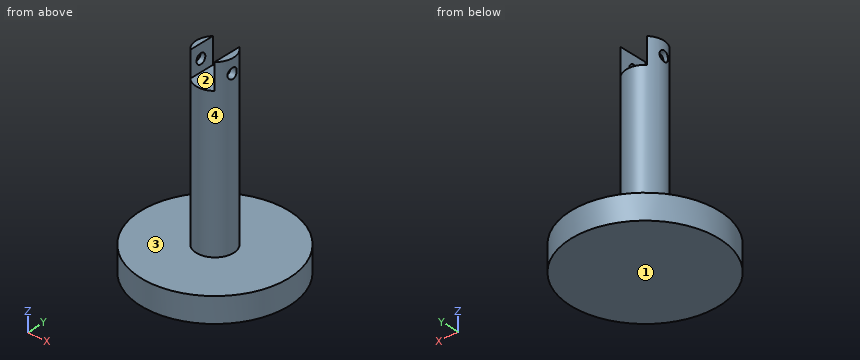
```python
from build123d import *

# Parameters (mm, degrees)
F0_R     = 75.4315959701
F1_DEPTH = 25.4
F10_R    = 19.05
F2_DEPTH = 203.2
F4_DEPTH = 26.25509
F5_R     = 5.3383463792
F6_DEPTH = 25.4
F7_R     = 5.1969918097
F8_DEPTH = 22.39609
F9_DEPTH = 72.38519


# Not quite as in the source:
# - a feature names something its author has since deleted; it is built from what else it names


with BuildPart() as f1:
    # F0 (on Top) → F1 (new body)
    with BuildSketch(Plane.XY):
        Circle(F0_R)
    extrude(amount=F1_DEPTH)

    # F10 (on Top) → F2 (join)
    with BuildSketch(Plane.XY):
        Circle(F10_R)
    extrude(amount=F2_DEPTH)

    # F3 (on face) → F4 (cut)
    with BuildSketch(Plane.XY.offset(203.2)):
        with BuildLine():
            ThreePointArc((12.2368524888, 14.6000664782), (-0.9386041951, 19.026863172), (-13.6144, 13.3248119176))
            Line((-13.6144, 13.3248119176), (-13.6144, -13.3248119176))
            ThreePointArc((-13.6144, -13.3248119176), (-0.9386041951, -19.026863172), (12.2368524888, -14.6000664782))
            Line((12.2368524888, -14.6000664782), (12.2368524888, 14.6000664782))
        make_face()
    extrude(amount=-F4_DEPTH, mode=Mode.SUBTRACT)

    # F5 (on face) → F6 (cut)
    with BuildSketch(Plane.YZ.offset(-13.6144)):
        with Locations((-189.9197250605, 0)):
            Circle(F5_R)
    extrude(amount=-F6_DEPTH, mode=Mode.SUBTRACT)

    # F7 (on face) → F8 (cut)
    with BuildSketch(Plane.YZ.offset(-13.6144)):
        with Locations((-0.8483366109, 189.2552375793)):
            Circle(F7_R)
    extrude(amount=-F8_DEPTH, mode=Mode.SUBTRACT)

    # F7 (on face) → F9 (cut)
    with BuildSketch(Plane.YZ.offset(-13.6144)):
        with Locations((-0.8483366109, 189.2552375793)):
            Circle(F7_R)
    extrude(amount=F9_DEPTH, mode=Mode.SUBTRACT)


solid = f1.part
```
Geometry: final body of the model. Coordinates: model frame, mm. Face numbers are marked on the shaded views. A direction names the side the tool comes from. Coordinates: 2 decimals unless noted, no trailing zeros. Order: outer loops, then holes, each group sorted by start corner. A loop starts at its lowest first (then second) coordinate and runs counter-clockwise, first axis right, second up. Notation, with made-up numbers: (68.25, -3) - (73.25, -3) arc R32 cw to (73.25, 29) - close; hole circle Ø1 at (-3.75, 10). An arc over 180 degrees is marked (long way). Write each question's results on one line, items separated by ' | '.
1) Section D-D, the plane y = 42. Return loops of the section in (x, z).
Results list:
outline: (-62.66, 0) - (62.66, 0) - (62.66, 25.4) - (-62.66, 25.4) - close
2) Pin query (flat end, axial travel): pin 1 (8 mm diameter, centred on y = 2, z = 195, fed in from +X); pin 2 (1 mm diameter, centred on x = -38, y = 8.5, fed in from -Z); pin 3 (12 mm diameter, centred on y = -0.85, z = 189.26, fed in from -X); pin 4 (6 mm diameter, centred on x = -55.5, y = 49.5, fed in from +Z). Return the tip coordinate at first contact, or that it passes through.
Results list:
pin 1: x = 19.05 | pin 2: z = 0 | pin 3: x = -19.05 | pin 4: z = 25.4
3) Set-up query: the marked faces 1 and 2. Return all of +Z, -Z, +X, -X, +Y, -Y with unobstructed straight access to the full face (end or side cutting, diameter ignored); none if empty.
Results list:
face 1: -Z, +X, -X, +Y, -Y | face 2: +Z, +Y, -Y
4) Section C-C, the plane z = 106. Return loops of the section in (x, y), plus the area to 3 significant figures.
Results list:
outline: circle Ø38.1 at (0, 0) | area: 1,140 mm^2
5) Line query: line 1 (Z direction, x = 44.5, y = 45); line 2 (Z direction, x = 7, y = -16.5); line 3 (X direction, y = 1, z = 102.5). Output: solid intervals per line, ascending. Write a range as from..to.
Results list:
line 1: 0..25.4 | line 2: 0..176.94 | line 3: -19.02..19.02
6) Pull-direction query (Y, two-part tool) for the marked faces 3 and 4; classes: pulls with the +Y half, pulls with the -Y half, needs draft (parallel to the pull), parting line crosses it, or undercut.
Results list:
face 3: needs draft | face 4: parting line crosses it
7) Section A-A, the plane y = 0. Return loops of the section in (x, z), plus the area to 3 significant figures.
Results list:
outline: (-75.43, 0) - (75.43, 0) - (75.43, 25.4) - (19.05, 25.4) - (19.05, 184.13) - (12.24, 184.13) - (12.24, 176.94) - (-13.61, 176.94) - (-13.61, 184.13) - (-19.05, 184.13) - (-19.05, 25.4) - (-75.43, 25.4) - close; (-19.05, 194.38) - (-13.61, 194.38) - (-13.61, 203.2) - (-19.05, 203.2) - close; (12.24, 194.38) - (19.05, 194.38) - (19.05, 203.2) - (12.24, 203.2) - close | area: 9,800 mm^2
8) Section B-B, the plane x = 0. Return loops of the section in (y, z), plus the area to 3 significant figures.
Results list:
outline: (-75.43, 0) - (75.43, 0) - (75.43, 25.4) - (19.05, 25.4) - (19.05, 176.94) - (-19.05, 176.94) - (-19.05, 25.4) - (-75.43, 25.4) - close | area: 9,610 mm^2
